Check sheet for the modelled part. Datum: model origin and axes. Units: mm. A direction names the side the tool comes from. Give positions to 0.01 mm unless a question says otherwise; leave off trailing zeros. Order: outer loops, then holes, each group sorted by start corner. A loop starts at its lowest first (then second) coordinate and runs counter-clockwise, first axis right, second up.
```python
from build123d import *

# Parameters (mm, degrees)
F0_W     = 100
F0_H     = 160
F1_DEPTH = 4
F2_W     = 4
F2_H     = 10
F3_DEPTH = 4


with BuildPart() as f1:
    # F0 (on Front) → F1 (new body)
    with BuildSketch(Plane.XZ):
        with Locations((50, 80)):
            Rectangle(F0_W, F0_H)
    extrude(amount=F1_DEPTH)

    # F2 (on face) → F3 (cut, through all)
    with BuildSketch(Plane.XZ.offset(4)):
        with Locations((2, 5)):
            Rectangle(F2_W, F2_H)
        with Locations((2, 25)):
            Rectangle(F2_W, F2_H)
        with Locations((2, 45)):
            Rectangle(F2_W, F2_H)
        with Locations((2, 65)):
            Rectangle(F2_W, F2_H)
        with Locations((2, 85)):
            Rectangle(F2_W, F2_H)
        with Locations((2, 105)):
            Rectangle(F2_W, F2_H)
        with Locations((2, 125)):
            Rectangle(F2_W, F2_H)
        with Locations((2, 145)):
            Rectangle(F2_W, F2_H)
        with Locations((98, 5)):
            Rectangle(F2_W, F2_H)
        with Locations((98, 125)):
            Rectangle(F2_W, F2_H)
        with Locations((98, 105)):
            Rectangle(F2_W, F2_H)
        with Locations((98, 145)):
            Rectangle(F2_W, F2_H)
        with Locations((98, 25)):
            Rectangle(F2_W, F2_H)
        with Locations((98, 65)):
            Rectangle(F2_W, F2_H)
        with Locations((98, 85)):
            Rectangle(F2_W, F2_H)
        with Locations((98, 45)):
            Rectangle(F2_W, F2_H)
    extrude(amount=-F3_DEPTH, mode=Mode.SUBTRACT)


solid = f1.part
```
(1) Set-up check for faces 4 (the face through (98, -2, 110)), 5 (the face through (2, -2, 50)), 6 (the face through (0, -2, 35)): record each of +Z, -Z, +X, -X, +Y, -Y from which the full face is reachable in a straight line by a thin tool's end or side.
Response values:
face 4: +X, +Y, -Y
face 5: -X, +Y, -Y
face 6: +Z, -Z, -X, +Y, -Y
(2) Release check for a two-part mould opening along Z. For faces 1 (the face through (2, -2, 90)), 2 (the face through (100, -2, 135)), 3 (the face through (2, -2, 80)) record: released by +Z, released by -Z, zero draft, split by the parting line, or undercut.
Response values:
face 1: undercut
face 2: zero draft
face 3: undercut
(3) Material ranges on L1, parallel to X at y = -0.2, z = 67.5, recorded low to high.
Response values:
L1: x = 4 to 96
(4) Gauge pin test, flat ends, axial feed: pin 1 Ø1.2 at (x, y) = (3, -2) entering from -Z; pin 2 Ø1.2 at (y, z) = (-2.5, 103) entering from +X; pin 3 Ø2 at (y, z) = (-1, 143.5) entering from -X. Record the tip position at first contact, or that the pin passes through.
Response values:
pin 1: stops at z = 10
pin 2: stops at x = 96
pin 3: stops at x = 4
(5) Cross-section at A-A on z = 143. Enter the section's corners in (x, y).
Response values:
outline: (4, -4) - (96, -4) - (96, 0) - (4, 0) - close
